Source: CAD feature listing. Evaluate the final solid. Frame: model axes, mm. Give positions to 0.01 mm unless a question says otherwise; leave off trailing zeros. Write each loop counter-clockwise with the first axis right and the second up, starting at its lowest first coordinate (ties: lowest second). Pieces come first, ordered by that corner, then holes. Notation, with made-up numbers: (49, 69) -> (71, 69) arc R9 cw to (71, 86) -> close; hole circle Ø3 at (53, -6). An arc over 180 degrees is marked (long way). Write item = value, one per line.
from build123d import *

# Parameters (mm, degrees)
CROQUIS1_W              = 240
CROQUIS1_H              = 500
CROQUIS1_R              = 5
SALIENTE_EXTRUIR1_DEPTH = 3
CROQUIS5_W              = 49.8
CROQUIS5_H              = 3
CROQUIS5_W_2            = 3
CROQUIS5_H_2            = 44.8
CORTAR_EXTRUIR2_DEPTH   = 4


with BuildPart() as part:
    # Croquis1 → Saliente-Extruir1 (new body)
    with BuildSketch(Plane.XY):
        Rectangle(CROQUIS1_W, CROQUIS1_H)
        with Locations((-80, -215)):
            Circle(CROQUIS1_R, mode=Mode.SUBTRACT)
        with Locations((80, -215)):
            Circle(CROQUIS1_R, mode=Mode.SUBTRACT)
        with Locations((80, 215)):
            Circle(CROQUIS1_R, mode=Mode.SUBTRACT)
        with Locations((-80, 215)):
            Circle(CROQUIS1_R, mode=Mode.SUBTRACT)
        with BuildLine():
            Line((-100, 201), (100, 201))
            ThreePointArc((100, 201), (104, 197), (100, 193))
            Line((100, 193), (-100, 193))
            ThreePointArc((-100, 193), (-104, 197), (-100, 201))
        make_face(mode=Mode.SUBTRACT)
        with BuildLine():
            Line((-100, 117), (100, 117))
            ThreePointArc((100, 117), (104, 121), (100, 125))
            Line((100, 125), (-100, 125))
            ThreePointArc((-100, 125), (-104, 121), (-100, 117))
        make_face(mode=Mode.SUBTRACT)
        with BuildLine():
            Line((-100, -111), (100, -111))
            ThreePointArc((100, -111), (104, -107), (100, -103))
            Line((100, -103), (-100, -103))
            ThreePointArc((-100, -103), (-104, -107), (-100, -111))
        make_face(mode=Mode.SUBTRACT)
        with BuildLine():
            Line((-100, -187), (100, -187))
            ThreePointArc((100, -187), (104, -183), (100, -179))
            Line((100, -179), (-100, -179))
            ThreePointArc((-100, -179), (-104, -183), (-100, -187))
        make_face(mode=Mode.SUBTRACT)
    extrude(amount=SALIENTE_EXTRUIR1_DEPTH)

    # Croquis5 → Cortar-Extruir2 (cut, through all)
    with BuildSketch(Plane(origin=(0, 0, 0), x_dir=(-1, 0, 0), z_dir=(0, 0, -1))):
        with Locations((-30, 248.5)):
            Rectangle(CROQUIS5_W, CROQUIS5_H)
        with Locations((70, 248.5)):
            Rectangle(CROQUIS5_W, CROQUIS5_H)
        with Locations((118.5, 180)):
            Rectangle(CROQUIS5_W_2, CROQUIS5_H_2)
        with Locations((118.5, 90)):
            Rectangle(CROQUIS5_W_2, CROQUIS5_H_2)
        with Locations((118.5, 0)):
            Rectangle(CROQUIS5_W_2, CROQUIS5_H_2)
        with Locations((118.5, -90)):
            Rectangle(CROQUIS5_W_2, CROQUIS5_H_2)
        with Locations((118.5, -180)):
            Rectangle(CROQUIS5_W_2, CROQUIS5_H_2)
        with Locations((70, -248.5)):
            Rectangle(CROQUIS5_W, CROQUIS5_H)
        with Locations((-30, -248.5)):
            Rectangle(CROQUIS5_W, CROQUIS5_H)
        with Locations((-118.5, -180)):
            Rectangle(CROQUIS5_W_2, CROQUIS5_H_2)
        with Locations((-118.5, -90)):
            Rectangle(CROQUIS5_W_2, CROQUIS5_H_2)
        with Locations((-118.5, 0)):
            Rectangle(CROQUIS5_W_2, CROQUIS5_H_2)
        with Locations((-118.5, 90)):
            Rectangle(CROQUIS5_W_2, CROQUIS5_H_2)
        with Locations((-118.5, 180)):
            Rectangle(CROQUIS5_W_2, CROQUIS5_H_2)
    extrude(amount=-CORTAR_EXTRUIR2_DEPTH, mode=Mode.SUBTRACT)


solid = part.part
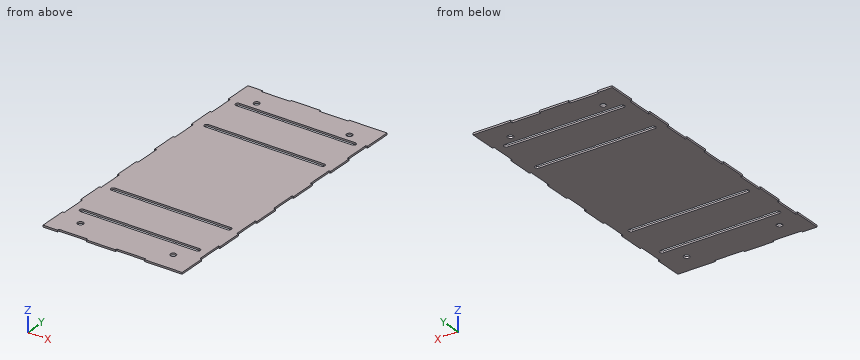
(1) Material intervals for line 1 (Y direction, x = 18.5, z = 1.3); line 2 (Y direction, x = 0, z = 2.55); line 3 (X direction, y = 177.5, z = 2.55), sorted ascending.
Values follow:
line_1 = -247 to -187, -179 to -111, -103 to 117, 125 to 193, 201 to 247
line_2 = -250 to -187, -179 to -111, -103 to 117, 125 to 193, 201 to 250
line_3 = -117 to 117
(2) Section query D-D (z = 1.5). Give the number of separate pieces and of enclosed holes in the cut face, plus the area to 3 significant figures.
Values follow:
separate_pieces = 1
enclosed_holes = 8
area = 111,000 mm2
(3) First-contact query: pin 1 (1.5 mm diameter, centred on y = -90, z = 1, fed in from -X); pin 2 (1.5 mm diameter, centred on x = 62.5, y = 119, fed in from -Z); pin 3 (1.5 mm diameter, centred on y = 179.5, z = 2, fed in from +X). Flat tips, straight axial feed; report the tip coordinate or a pass-through.
Values follow:
pin_1 = -117
pin_2 = through
pin_3 = 117
(4) Section query B-B (x = -14.5). Return loops of the section in (y, z), plus the area to 3 significant figures.
Values follow:
outline = (-250, 0) -> (-187, 0) -> (-187, 3) -> (-250, 3) -> close; (-179, 0) -> (-111, 0) -> (-111, 3) -> (-179, 3) -> close; (-103, 0) -> (117, 0) -> (117, 3) -> (-103, 3) -> close; (125, 0) -> (193, 0) -> (193, 3) -> (125, 3) -> close; (201, 0) -> (250, 0) -> (250, 3) -> (201, 3) -> close
area = 1,400 mm2
(5) Section query C-C (x = 34.5). Return loops of the section in (y, z), plus the area to 3 significant figures.
Values follow:
outline = (-247, 0) -> (-187, 0) -> (-187, 3) -> (-247, 3) -> close; (-179, 0) -> (-111, 0) -> (-111, 3) -> (-179, 3) -> close; (-103, 0) -> (117, 0) -> (117, 3) -> (-103, 3) -> close; (125, 0) -> (193, 0) -> (193, 3) -> (125, 3) -> close; (201, 0) -> (247, 0) -> (247, 3) -> (201, 3) -> close
area = 1,390 mm2
(6) Section query A-A (y = -215). Return loops of the section in (x, z).
Values follow:
outline = (-120, 0) -> (-85, 0) -> (-85, 3) -> (-120, 3) -> close; (-75, 0) -> (75, 0) -> (75, 3) -> (-75, 3) -> close; (85, 0) -> (120, 0) -> (120, 3) -> (85, 3) -> close
